Can you work these out from the model? Positions are in its coordinate system, mm. Coordinates: 2 decimals unless noted, no trailing zeros. Order: outer loops, then holes, each group sorted by start corner. A loop starts at its lowest first (then second) coordinate and runs counter-clockwise, first axis right, second up. Notation, with made-up numbers: (-5.5, 3.25) -> (21.5, 3.25) arc R10 cw to (21.5, 19.25) -> close; hole circle Ø7 at (87.5, 70). An arc over 180 degrees is marked (long way). Return JSON: item names as keys, results as strings. Group by question number.
1) If we section it at D-D, the plane z = 63.5: Please give me the cut outline in (x, y), then the cut area to 3 significant figures.
2) If we section it at C-C, the plane y = 2.15: State how many separate pieces and enclosed holes the cut face has, then the cut area to 3 significant figures.
3) For pin 1 (3 mm diameter, centred on y = 4, z = 54, fed in from +X); pin 2 (1.5 mm diameter, centred on x = 9.5, y = 1.5, fed in from +Z); pin 3 (2 mm diameter, centred on y = 1.5, z = 21.5, fed in from -X), each with a flat end and sliding along its axis, tell me the tip position at first contact or that it passes through.
4) If I drill on probe 1 along X at (y, z) = (2.7, -26.5); probe 2 along X at (y, z) = (4.8, -8); probe 3 along Z at (x, y) = (2, 3.15), over which ranges is the centre line in solid material (lowest first)? Write a range as from..to.
5) If we section it at B-B, the plane x = -40: Please give me the cut outline in (y, z).
6) If we section it at A-A, the plane z = 45: Please give me the cut outline in (x, y).
from build123d import *

# Parameters (mm, degrees)
SKETCH1_R           = 72.5
BOSS_EXTRUDE1_DEPTH = 5
CUT_EXTRUDE6_REACH  = 104.652
SKETCH7_R           = 2
CIRPATTERN1_COUNT   = 3


with BuildPart() as part:
    # Sketch1 → Boss-Extrude1 (new body)
    with BuildSketch(Plane(origin=(0, 0, 0), x_dir=(1, 0, 0), z_dir=(0, 1, 0))):
        with Locations(Location((0, 0, 0), (0, 0, 270))):
            Circle(SKETCH1_R)
    extrude(amount=BOSS_EXTRUDE1_DEPTH)

    # Sketch7 → Cut-Extrude6 (cut, up to next)
    with BuildSketch(Plane(origin=(0, 5, 0), x_dir=(1, 0, 0), z_dir=(0, 1, 0)), mode=Mode.PRIVATE) as cut_extrude6_sk1:
        with Locations(Location((15, 48.062177826, 0), (0, 0, 270))):
            Circle(SKETCH7_R)
    cut_extrude6_tool1 = extrude(cut_extrude6_sk1.sketch, amount=-CUT_EXTRUDE6_REACH, mode=Mode.PRIVATE) & part.part
    # Sketch7 → Cut-Extrude6 (cut, up to next)
    with BuildSketch(Plane(origin=(0, 5, 0), x_dir=(1, 0, 0), z_dir=(0, 1, 0)), mode=Mode.PRIVATE) as cut_extrude6_sk2:
        with Locations(Location((18.5, 42, 0), (0, 0, 270))):
            Circle(SKETCH7_R)
    cut_extrude6_tool2 = extrude(cut_extrude6_sk2.sketch, amount=-CUT_EXTRUDE6_REACH, mode=Mode.PRIVATE) & part.part
    # Sketch7 → Cut-Extrude6 (cut, up to next)
    with BuildSketch(Plane(origin=(0, 5, 0), x_dir=(1, 0, 0), z_dir=(0, 1, 0)), mode=Mode.PRIVATE) as cut_extrude6_sk3:
        with Locations(Location((-22.672105065, 26.312177826, 0), (0, 0, 270))):
            Circle(SKETCH7_R)
    cut_extrude6_tool3 = extrude(cut_extrude6_sk3.sketch, amount=-CUT_EXTRUDE6_REACH, mode=Mode.PRIVATE) & part.part
    # Sketch7 → Cut-Extrude6 (cut, up to next)
    with BuildSketch(Plane(origin=(0, 5, 0), x_dir=(1, 0, 0), z_dir=(0, 1, 0)), mode=Mode.PRIVATE) as cut_extrude6_sk4:
        with Locations(Location((-19.172105065, 20.25, 0), (0, 0, 270))):
            Circle(SKETCH7_R)
    cut_extrude6_tool4 = extrude(cut_extrude6_sk4.sketch, amount=-CUT_EXTRUDE6_REACH, mode=Mode.PRIVATE) & part.part
    # Sketch7 → Cut-Extrude6 (cut, up to next)
    with BuildSketch(Plane(origin=(0, 5, 0), x_dir=(1, 0, 0), z_dir=(0, 1, 0)), mode=Mode.PRIVATE) as cut_extrude6_sk5:
        with Locations(Location((32.965163285, 58.902869281, 0), (0, 0, 270))):
            Circle(SKETCH7_R)
    cut_extrude6_tool5 = extrude(cut_extrude6_sk5.sketch, amount=-CUT_EXTRUDE6_REACH, mode=Mode.PRIVATE) & part.part
    # Sketch7 → Cut-Extrude6 (cut, up to next)
    with BuildSketch(Plane(origin=(0, 5, 0), x_dir=(1, 0, 0), z_dir=(0, 1, 0)), mode=Mode.PRIVATE) as cut_extrude6_sk6:
        Polygon((26.486526778, 28.135814771), (44.240047555, 38.385814771), (47.490047555, 32.756649646), (29.736526778, 22.506649646), align=None)
    cut_extrude6_tool6 = extrude(cut_extrude6_sk6.sketch, amount=-CUT_EXTRUDE6_REACH, mode=Mode.PRIVATE) & part.part
    cut_extrude6_1 = cut_extrude6_tool1.solids().sort_by_distance((15, 5, -48.062178))[0]
    add(cut_extrude6_1, mode=Mode.SUBTRACT)
    cut_extrude6_2 = cut_extrude6_tool2.solids().sort_by_distance((18.5, 5, -42))[0]
    add(cut_extrude6_2, mode=Mode.SUBTRACT)
    cut_extrude6_3 = cut_extrude6_tool3.solids().sort_by_distance((-22.672105, 5, -26.312178))[0]
    add(cut_extrude6_3, mode=Mode.SUBTRACT)
    cut_extrude6_4 = cut_extrude6_tool4.solids().sort_by_distance((-19.172105, 5, -20.25))[0]
    add(cut_extrude6_4, mode=Mode.SUBTRACT)
    cut_extrude6_5 = cut_extrude6_tool5.solids().sort_by_distance((32.965163, 5, -58.902869))[0]
    add(cut_extrude6_5, mode=Mode.SUBTRACT)
    cut_extrude6_6 = cut_extrude6_tool6.solids().sort_by_distance((36.988287, 5, -30.446232))[0]
    add(cut_extrude6_6, mode=Mode.SUBTRACT)
    cut_extrude6 = cut_extrude6_1 + cut_extrude6_2 + cut_extrude6_3 + cut_extrude6_4 + cut_extrude6_5 + cut_extrude6_6  # Cut-Extrude6 as one shape, for the pattern or mirror that repeats it

    # CirPattern1: Cut-Extrude6 ×3 about axis
    cirpattern1_axis = Axis((0, 0, 0), (0, 1, 0))
    for i in range(1, CIRPATTERN1_COUNT):
        add(cut_extrude6.rotate(cirpattern1_axis, i * 360 / CIRPATTERN1_COUNT), mode=Mode.SUBTRACT)


solid = part.part
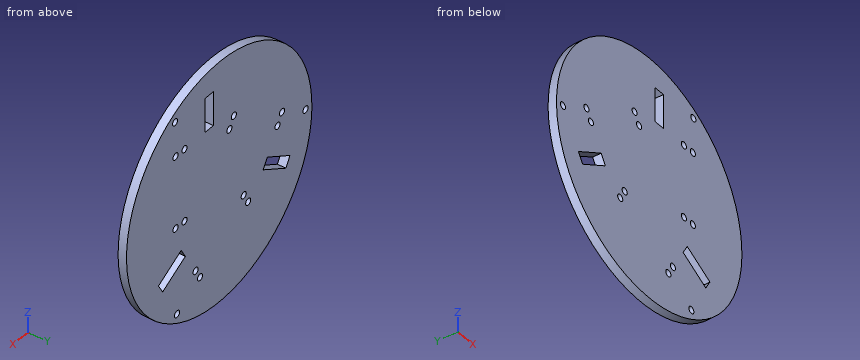
Result sheet:
{
 "1": {"outline": "(-34.99, 0) -> (34.99, 0) -> (34.99, 5) -> (-34.99, 5) -> close", "area": "350 mm2"},
 "2": {"separate pieces": "1", "enclosed holes": "18", "area": "15,900 mm2"},
 "3": {"pin 1": "stops at x = 50", "pin 2": "stops at z = 71.97", "pin 3": "stops at x = -69.54"},
 "4": {"probe 1": "x = -67.48..-24.66, -20.68..27.43, 36.65..67.48", "probe 2": "x = -72.06..25.82, 28.42..32.82, 35.42..72.06", "probe 3": "z = -72.47..72.47"},
 "5": {"outline": "(0, -60.47) -> (5, -60.47) -> (5, -17.76) -> (0, -17.76) -> close; (0, -10.25) -> (5, -10.25) -> (5, 60.47) -> (0, 60.47) -> close"},
 "6": {"outline": "(-56.84, 0) -> (4.62, 0) -> (4.62, 5) -> (-56.84, 5) -> close; (11.12, 0) -> (56.84, 0) -> (56.84, 5) -> (11.12, 5) -> close"}
}
